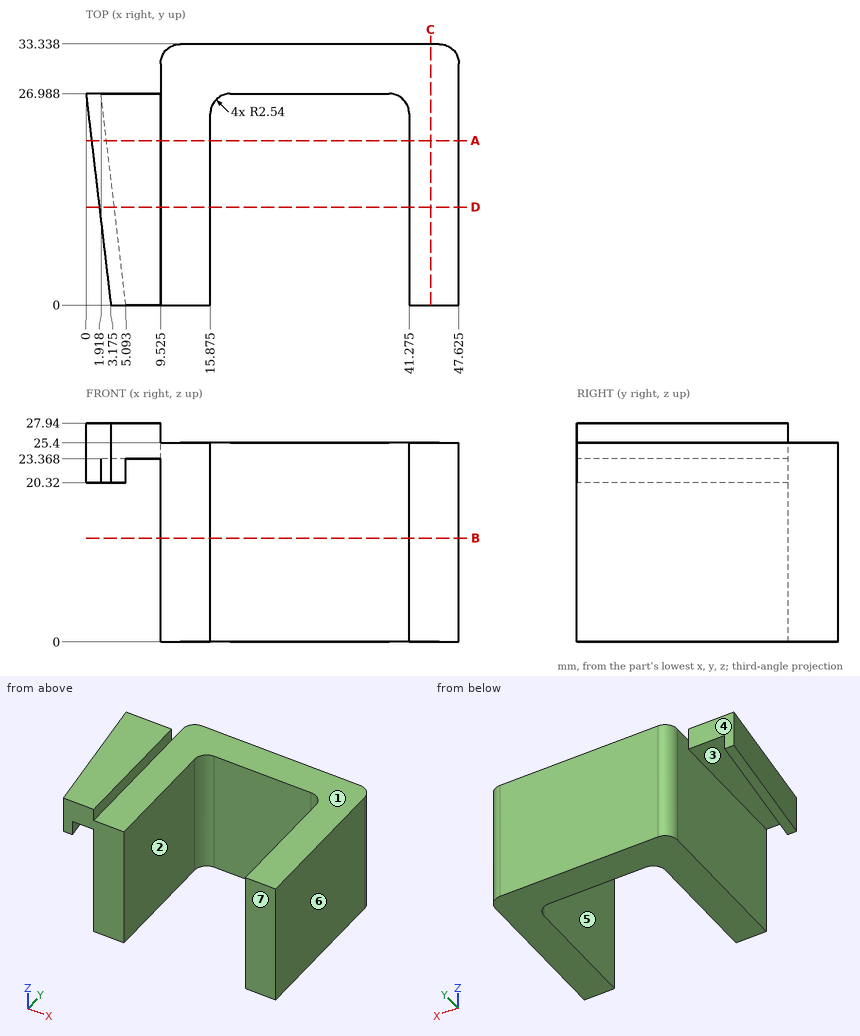
The drawing under review shows one solid part. Ordinate dimensions are in mm from its lowest x, y, z. A direction names the side the tool comes from. Give positions to 0.01 mm unless a question says otherwise; leave off trailing zeros. Write each loop counter-clockwise with the first axis right and the second up, starting at its lowest first coordinate (ties: lowest second). Pieces come first, ordered by that corner, then holes.
1. Add section A-A, the plane y = 21. Write out the cut boundary in (x, z) (1 decimal).
2. Add section B-B, the plane z = 13.25. Write out the cut boundary in (x, y) (1 decimal).
3. Tool access review of the marked faces 1, 2, 3 and 4: name each direction out of +Z, -Z, +X, -X, +Y, -Y from which nothing blocks a thin tool from reaching the whole face with its end or side.
4. Wall thickness on L1, parallel to X at y = 23, z = 20.5 (1 decimal); L2, parallel to X at y = 8, z = 13.5 (1 decimal); L3, parallel to X at y = 26.5, z = 22.5 (1 decimal): over which ranges is each line inside the solid? List them lowest first.
5. Draft analysis for pull direction X (two halves, no side actions). For the marked faces 5, 6 and 7, state which applies: +X half, -X half, draft (parallel to the pull), parting line (faces both ways), or undercut.
6. Add section C-C, the plane x = 44. Write out the cut boundary in (y, z).
7. Add section D-D, the plane y = 12.5. Write out the cut boundary in (x, z) (1 decimal).
8. For P1, Ø12, axis at y = 7.5, z = 12.5, coming from the -X side (1 decimal); P2, Ø8, axis at x = 19, z = 7.5, coming from the -Y side; P3, Ø2.5, axis at x = 6.5, z = 23.5, coming from the +Y side; P4, Ø2, axis at y = 11, z = 27, coming from the +X side (1 decimal), all flat-tipped, find the tip position at first contact; note any pin that passes through.
Worked answers:
1. outline: (0.7, 20.3) - (2.6, 20.3) - (2.6, 23.4) - (9.5, 23.4) - (9.5, 0) - (15.9, 0) - (15.9, 25.4) - (9.5, 25.4) - (9.5, 27.9) - (0.7, 27.9) - close; (41.3, 0) - (47.6, 0) - (47.6, 25.4) - (41.3, 25.4) - close
2. outline: (9.5, 0) - (15.9, 0) - (15.9, 24.4) arc R2.5 cw to (18.4, 27) - (38.7, 27) arc R2.5 cw to (41.3, 24.4) - (41.3, 0) - (47.6, 0) - (47.6, 30.8) arc R2.5 ccw to (45.1, 33.3) - (12.1, 33.3) arc R2.5 ccw to (9.5, 30.8) - close
3. face 1: +Z, +X, +Y, -Y
3. face 2: +Z, -Z, -Y
3. face 3: -Z, +Y
3. face 4: +Z, -Z, -X, +Y
4. L1: x = 0.5 to 2.4, 9.5 to 15.9, 41.3 to 47.6
4. L2: x = 9.5 to 15.9, 41.3 to 47.6
4. L3: x = 0.1 to 2, 9.5 to 16.9, 40.2 to 47.6
5. face 5: undercut
5. face 6: +X half
5. face 7: draft
6. outline: (0, 0) - (33.34, 0) - (33.34, 25.4) - (0, 25.4) - close
7. outline: (1.7, 20.3) - (3.6, 20.3) - (3.6, 23.4) - (9.5, 23.4) - (9.5, 0) - (15.9, 0) - (15.9, 25.4) - (9.5, 25.4) - (9.5, 27.9) - (1.7, 27.9) - close; (41.3, 0) - (47.6, 0) - (47.6, 25.4) - (41.3, 25.4) - close
8. P1: stops at x = 9.5
8. P2: stops at y = 0
8. P3: stops at y = 26.99
8. P4: stops at x = 9.5
